Model file for the job. Use its own axes, mm. A direction names the side the tool comes from. Round coordinates to 2 decimals unless told otherwise and drop trailing zeros. Loops run counter-clockwise (first coordinate to the right, second up) from the corner with the lowest first, then second, coordinate; pieces in that order, holes last. Notation, with made-up numbers: (59, 6.25) -> (66, 6.25) arc R18 ccw to (66, 30.25) -> close; hole circle Ø2 at (86.25, -20.75). An arc over 180 degrees is marked (long way). Use a Markdown table: item, result.
from build123d import *

# Parameters (mm, degrees)
SKETCH1_W           = 108
SKETCH1_H           = 108
SKETCH1_R           = 6
SKETCH1_R_2         = 15
BOSS_EXTRUDE1_DEPTH = 14
SKETCH2_R           = 20
SKETCH2_R_2         = 15
BOSS_EXTRUDE2_DEPTH = 26.2
SKETCH3_R           = 41.5
SKETCH3_R_2         = 15
BOSS_EXTRUDE3_DEPTH = 17


with BuildPart() as part:
    # Sketch1 → Boss-Extrude1 (new body)
    with BuildSketch(Plane(origin=(0, 0, 0), x_dir=(1, 0, 0), z_dir=(0, 1, 0))):
        with Locations((54, 54)):
            Rectangle(SKETCH1_W, SKETCH1_H)
        with Locations(Location((12.75, 12.75, 0), (0, 0, 270))):
            Circle(SKETCH1_R, mode=Mode.SUBTRACT)
        with Locations(Location((54, 54, 0), (0, 0, 270))):
            Circle(SKETCH1_R_2, mode=Mode.SUBTRACT)
        with Locations(Location((95.25, 12.75, 0), (0, 0, 270))):
            Circle(SKETCH1_R, mode=Mode.SUBTRACT)
        with Locations(Location((95.25, 95.25, 0), (0, 0, 270))):
            Circle(SKETCH1_R, mode=Mode.SUBTRACT)
        with Locations(Location((12.75, 95.25, 0), (0, 0, 270))):
            Circle(SKETCH1_R, mode=Mode.SUBTRACT)
    extrude(amount=BOSS_EXTRUDE1_DEPTH)

    # Sketch2 → Boss-Extrude2 (add)
    with BuildSketch(Plane(origin=(0, 14, 0), x_dir=(1, 0, 0), z_dir=(0, 1, 0))):
        with Locations(Location((54, 54, 0), (0, 0, 90))):
            Circle(SKETCH2_R)
        with Locations(Location((54, 54, 0), (0, 0, 270))):
            Circle(SKETCH2_R_2, mode=Mode.SUBTRACT)
    extrude(amount=BOSS_EXTRUDE2_DEPTH)

    # Sketch3 → Boss-Extrude3 (add)
    with BuildSketch(Plane(origin=(0, 14, 0), x_dir=(1, 0, 0), z_dir=(0, 1, 0))):
        with Locations(Location((54, 54, 0), (0, 0, 90))):
            Circle(SKETCH3_R)
        with Locations(Location((54, 54, 0), (0, 0, 270))):
            Circle(SKETCH3_R_2, mode=Mode.SUBTRACT)
    extrude(amount=BOSS_EXTRUDE3_DEPTH)


solid = part.part
Q1. Band-saw the part on B-B, the plane y = 5.5. Give the cut face in (x, z), plus the area to 3 significant figures.
Results list:
| item | result |
|---|---|
| outline | (0, -108) -> (108, -108) -> (108, 0) -> (0, 0) -> close; hole circle Ø12 at (12.75, -95.25); hole circle Ø12 at (12.75, -12.75); hole circle Ø30 at (54, -54); hole circle Ø12 at (95.25, -95.25); hole circle Ø12 at (95.25, -12.75) |
| area | 10,500 mm² |
Q2. Band-saw the part on D-D, the plane y = 29.5. Give the cut face in (x, z), plus the area to 3 significant figures.
Results list:
| item | result |
|---|---|
| outline | circle Ø83 at (54, -54); hole circle Ø30 at (54, -54) |
| area | 4,700 mm² |
Q3. Band-saw the part on A-A, the plane z = -54. Give the cut face in (x, y).
Results list:
| item | result |
|---|---|
| outline | (0, 0) -> (39, 0) -> (39, 40.2) -> (34, 40.2) -> (34, 31) -> (12.5, 31) -> (12.5, 14) -> (0, 14) -> close; (69, 0) -> (108, 0) -> (108, 14) -> (95.5, 14) -> (95.5, 31) -> (74, 31) -> (74, 40.2) -> (69, 40.2) -> close |
Q4. Flat gauge pins, fed straight in: pin 1 (5 mm diameter, centred on x = 53, y = 18.5, fed in from -Z); pin 2 (6 mm diameter, centred on x = 62, z = -88, fed in from +Y); pin 3 (19 mm diameter, centred on x = 95.25, z = -12.75, fed in from +Y); pin 4 (9.5 mm diameter, centred on x = 12.75, z = -95.25, fed in from +Y). Where does each tip first touch, or does it go through?
Results list:
| item | result |
|---|---|
| pin 1 | stops at z = -95.5 |
| pin 2 | stops at y = 31 |
| pin 3 | stops at y = 14 |
| pin 4 | passes through |
Q5. Drill centre lines: L1, parallel to X at y = 4.75, z = -12.75; L2, parallel to Z at x = 95, y = 5; L3, parallel to X at y = 33, z = -54. Where is each one in solid material? Low to high. Write a range as from..to.
Results list:
| item | result |
|---|---|
| L1 | x = 0..6.75, 18.75..89.25, 101.25..108 |
| L2 | z = -108..-101.24, -89.26..-18.74, -6.76..0 |
| L3 | x = 34..39, 69..74 |
Q6. Tool access for faces 1 (the face through (44, 31, -72)), 2 (the face through (100.309, 6.902, -9.524)): list every direction of +Z, -Z, +X, -X, +Y, -Y with a clear straight run to the whole face (end or side of a thin tool).
Results list:
| item | result |
|---|---|
| face 1 | +Y |
| face 2 | +Y, -Y |
Q7. Band-saw the part on C-C, the plane z = -83. Give the cut face in (x, y), plus the area to 3 significant figures.
Results list:
| item | result |
|---|---|
| outline | (0, 0) -> (108, 0) -> (108, 14) -> (83.69, 14) -> (83.69, 31) -> (24.31, 31) -> (24.31, 14) -> (0, 14) -> close |
| area | 2,520 mm² |
Q8. Pull direction Z, two halves, no side cores. Call faces 3 (the face through (64.138, 19.819, -65.056)), 4 (the face through (39, 40.2, -57)), 5 (the face through (53, 7, 0)): released by +Z, released by -Z, zero draft, split by the parting line, or undercut.
Results list:
| item | result |
|---|---|
| face 3 | undercut |
| face 4 | zero draft |
| face 5 | released by +Z |
